Verification items for the finished model (mm, model axes). Round coordinates to 2 decimals unless told otherwise and drop trailing zeros. Order: outer loops, then holes, each group sorted by start corner. A loop starts at its lowest first (then second) coordinate and runs counter-clockwise, first axis right, second up. Notation, with made-up numbers: (21.25, -27.75) -> (49.25, -27.75) arc R21 cw to (49.25, -7.75) -> close; hole circle Ø1 at (-19, 42). An arc over 180 degrees is marked (long way). Return JSON: item names as keys, results as strings. Group by question number.
1) Section check A-A on x = -55. Enter the section's corners in (y, z), plus the area to 3 significant figures.
2) Section check D-D on y = 90. Enter the section's corners in (x, z), plus the area to 3 significant figures.
3) Section check C-C on x = 25. Enter the section's corners in (y, z), plus the area to 3 significant figures.
4) Section check B-B on z = 3.05. State how many separate pieces and enclosed holes the cut face has, plus the area to 3 significant figures.
5) Scan lines: L1, parallel to Y at x = 0, z = 3.05; L2, parallel to X at y = -105.3, z = 1.2; L3, parallel to X at y = 74, z = 0.85. Record each from-to range of solid material in increasing order.
6) Depth check by flat-ended pin: pin 1 (5 mm diameter, centred on x = 21.5, y = -56.5, fed in from -Z); pin 2 (2.5 mm diameter, centred on x = 49, z = 2.5, fed in from +Y); pin 3 (3 mm diameter, centred on x = 0, y = -83.3, fed in from -Z); pin 4 (2 mm diameter, centred on x = -40.5, z = 2, fed in from -Y). Enter the tip coordinate at first touch or a pass-through.
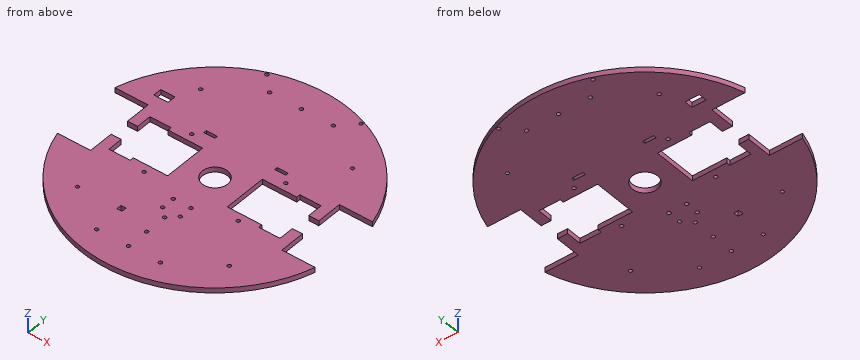
Autodesk Fusion 360 part; units mm, degrees
sketch "Sketch1" plane through (0, 0, 0) normal (0, 0, 1) x (1, 0, 0)
  circle A0 centre (0, 0) radius 132
  line L0 (-29.5, 21.3) -> (-29.5, -21.3)
  line L1 (-94.5, -35) -> (-127.2753, -35)
  line L2 (-63.5, 21.3) -> (-29.5, 21.3)
  line L3 (-63.5, -21.3) -> (-29.5, -21.3)
  line L4 (-63.5, 25) -> (-84.5, 25)
  line L5 (-84.5, -25) -> (-63.5, -25)
  line L6 (-63.5, -25) -> (-63.5, -21.3)
  line L7 (-63.5, 21.3) -> (-63.5, 25)
  line L8 (-94.5, 35) -> (-127.2753, 35)
  circle A1 centre (-46.5, 29) radius 1.75
  circle A2 centre (-46.5, -29) radius 1.75
  line L9 (0, 2.5) -> (0, 20)
  circle A3 centre (8.75, -53) radius 1.75
  circle A4 centre (8.75, -40) radius 1.75
  circle A5 centre (-8.75, -40) radius 1.75
  circle A6 centre (-8.75, -53) radius 1.75
  line L10 (-124.5, -35) -> (-124.5, 35)
  line L11 (-84.5, -10) -> (-94.5, -10)
  line L12 (-84.5, 10) -> (-94.5, 10)
  line L13 (-84.5, 25) -> (-84.5, 10)
  line L14 (-84.5, -10) -> (-84.5, -25)
  line L15 (-94.5, -35) -> (-94.5, -10)
  line L16 (-94.5, 10) -> (-94.5, 35)
  line L17 (94.5, -35) -> (94.5, -10)
  line L18 (94.5, 10) -> (94.5, 35)
  circle A7 centre (46.5, 29) radius 1.75
  line L19 (63.5, 25) -> (84.5, 25)
  line L20 (94.5, 35) -> (127.2753, 35)
  line L21 (84.5, 25) -> (84.5, 10)
  line L22 (29.5, 21.3) -> (29.5, -21.3)
  line L23 (84.5, -10) -> (94.5, -10)
  line L24 (124.5, -35) -> (124.5, 35)
  line L25 (63.5, -25) -> (63.5, -21.3)
  line L26 (84.5, -10) -> (84.5, -25)
  line L27 (84.5, -25) -> (63.5, -25)
  line L28 (63.5, -21.3) -> (29.5, -21.3)
  line L29 (63.5, 21.3) -> (29.5, 21.3)
  line L30 (94.5, -35) -> (127.2753, -35)
  circle A8 centre (46.5, -29) radius 1.75
  line L31 (84.5, 10) -> (94.5, 10)
  line L32 (63.5, 21.3) -> (63.5, 25)
  line L33 (40.5, 36.3) -> (29.5, 36.3)
  line L34 (29.5, 36.3) -> (29.5, 39.3)
  line L35 (29.5, 39.3) -> (40.5, 39.3)
  line L36 (40.5, 39.3) -> (40.5, 36.3)
  line L37 (-40.5, 39.3) -> (-40.5, 36.3)
  line L38 (-40.5, 36.3) -> (-29.5, 36.3)
  line L39 (-29.5, 39.3) -> (-40.5, 39.3)
  line L40 (-29.5, 36.3) -> (-29.5, 39.3)
  line L41 (-84.5, 47) -> (-98.5, 47)
  line L42 (-98.5, 47) -> (-98.5, 55.4)
  line L43 (-98.5, 55.4) -> (-84.5, 55.4)
  line L44 (-84.5, 55.4) -> (-84.5, 47)
  circle A9 centre (0, -105.3) radius 1.75
  circle A10 centre (0, -83.3) radius 1.75
  circle A11 centre (0, -61.3) radius 1.75
  line L45 (-30, -76.3) -> (-35, -76.3)
  line L46 (-35, -76.3) -> (-35, -71.3)
  line L47 (-35, -71.3) -> (-30, -71.3)
  line L48 (-30, -71.3) -> (-30, -76.3)
  circle A12 centre (75, -75) radius 1.75
  circle A13 centre (75, 75) radius 1.75
  circle A14 centre (-75, 75) radius 1.75
  circle A15 centre (-75, -75) radius 1.75
  circle A16 centre (-31.5, -105.3) radius 1.75
  circle A17 centre (31.5, -105.3) radius 1.75
  circle A18 centre (-31.5, 105.3) radius 1.75
  circle A19 centre (31.5, 105.3) radius 1.75
  circle A20 centre (0, 105.3) radius 1.75
  circle A21 centre (-46.5, 120.5) radius 1.75
  circle A22 centre (46.5, 120.5) radius 1.75
  circle A23 centre (0, 0) radius 12.5
  point P0 (0, 80.767)
  point P1 (0, -132)
  point P2 (0, -83.3)
  point P3 (0, 74)
  dimension "d1" = 264
  dimension "d12" = 42.6
  dimension "d14" = 21.3
  dimension "d15" = 21
  dimension "d16" = 50
  dimension "d20" = 34
  dimension "d24" = 3.7
  dimension "d25" = 3.7
  dimension "d28" = 10
  dimension "d30" = 3.5
  dimension "d31" = 7.7
  dimension "d32" = 17
  dimension "d33" = 7.7
  dimension "d34" = 17
  dimension "d111" = 40
  dimension "d112" = 30
  dimension "d113" = 15
  dimension "d114" = 15
  dimension "d119" = 3.5
  dimension "d124" = 3.5
  dimension "d127" = 13
  dimension "d129" = 3.5
  dimension "d130" = 11
  dimension "d131" = 3
  dimension "d134" = 70
  dimension "d148" = 8.4
  dimension "d150" = 3.5
  dimension "d151" = 3.5
  dimension "d153" = 22
  dimension "d154" = 3.5
  dimension "d155" = 22
  dimension "d160" = 5
  dimension "d161" = 5
  dimension "d162" = 30
  dimension "d163" = 10
  dimension "d164" = 3.5
  dimension "d190" = 3.5
  dimension "d191" = 3.5
  dimension "d209" = 13
  dimension "d211" = 31.5
  dimension "d212" = 31.5
  dimension "d220" = 29.5
  dimension "d221" = 29.5
  dimension "d222" = 12
  dimension "d223" = 14
  dimension "d224" = 10
  dimension "d226" = 15
  dimension "d229" = 18.7
  dimension "d236" = 50
  dimension "d237" = 19.5
  dimension "d238" = 50
  dimension "d239" = 19.5
  dimension "d240" = 3.5
  dimension "d242" = 91.5
  dimension "d243" = 3.5
  dimension "d244" = 3.5
  dimension "d245" = 9.5
  dimension "d246" = 19.6
  dimension "d247" = 3.5
  dimension "d248" = 40
  dimension "d249" = 19.5
  dimension "d250" = 3.5
  dimension "d251" = 25
  dimension "d253" = 46.5
  dimension "d255" = 91.5
  dimension "d256" = 40
  dimension "d261" = 8.75
  dimension "d262" = 8.75
  dimension "d263" = 13
  dimension "d264" = 8.75
  dimension "d265" = 17.5
  dimension "d266" = 8.3
  dimension "d267" = 8.75
  dimension "d268" = 29
  dimension "d269" = 3.5
  dimension "d270" = 22
extrude "Extrude1" add sketch "Sketch1" along normal blind 5 contours A0 L0 L1 L2 L3 L4 L5 L6 L7 L8 L11 L12 L13 L14 L15 L16 L17 L18 L19 L20 L21 L22 L23 L25 L26 L27 L28 L29 L30 L31 L32
Check result:
{
 "1": {"outline": "(-120, 0) -> (-21.3, 0) -> (-21.3, 5) -> (-120, 5) -> close; (21.3, 0) -> (120, 0) -> (120, 5) -> (21.3, 5) -> close", "area": "987 mm^2"},
 "2": {"outline": "(-96.56, 0) -> (96.56, 0) -> (96.56, 5) -> (-96.56, 5) -> close", "area": "966 mm^2"},
 "3": {"outline": "(-129.61, 0) -> (129.61, 0) -> (129.61, 5) -> (-129.61, 5) -> close", "area": "1,300 mm^2"},
 "4": {"separate pieces": "1", "enclosed holes": "27", "area": "43,400 mm^2"},
 "5": {"L1": "-132 to -107.05, -103.55 to -85.05, -81.55 to -63.05, -59.55 to -12.5, 12.5 to 103.55, 107.05 to 132", "L2": "-79.6 to -33.25, -29.75 to -1.75, 1.75 to 29.75, 33.25 to 79.6", "L3": "-109.31 to -76.44, -73.56 to 73.56, 76.44 to 109.31"},
 "6": {"pin 1": "z = 0", "pin 2": "y = 123.06", "pin 3": "through", "pin 4": "y = -125.95"}
}
